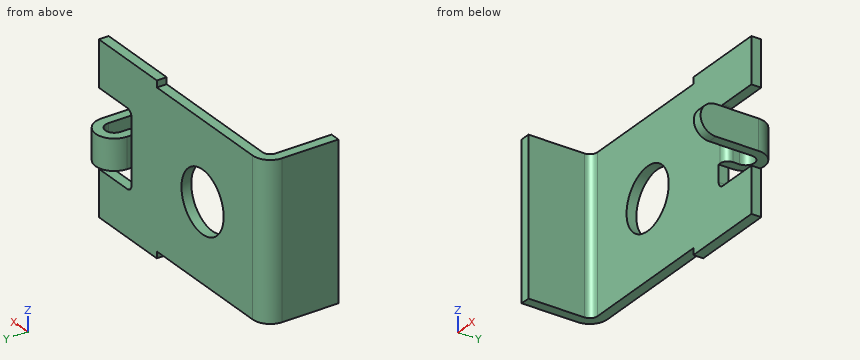
```python
from build123d import *

# Parameters (mm, degrees)
EXTRUDE_THIN1_DEPTH = 6.4135
SKETCH2_W           = 6.985
SKETCH2_H           = 0.8128
BOSS_EXTRUDE1_DEPTH = 6.9596
SKETCH3_W           = 3.937
SKETCH3_H           = 6.35
CUT_EXTRUDE1_DEPTH  = 23.027014146
EXTRUDE_THIN2_DEPTH = 1.27
FILLET1_RADIUS      = 1.27
FILLET1_LENGTH      = 0.8128
FILLET2_R           = 0.635
SKETCH5_R           = 2.54
CUT_EXTRUDE2_DEPTH  = 23.027014146
FILLET3_R           = 0.508


with BuildPart() as part:
    # Sketch1 → Extrude-Thin1 (new, symmetric)
    with BuildSketch(Plane.XY):
        with BuildLine():
            Line((0, 0), (0, 4.6482))
            ThreePointArc((0, 4.6482), (0.424050802, 5.671949198), (1.4478, 6.096))
            Line((1.4478, 6.096), (19.9898, 6.096))
            Line((19.9898, 6.096), (19.9898, 5.2832))
            Line((19.9898, 5.2832), (1.4478, 5.2832))
            ThreePointArc((1.4478, 5.2832), (0.998787194, 5.097212806), (0.8128, 4.6482))
            Line((0.8128, 4.6482), (0.8128, 0))
            Line((0.8128, 0), (0, 0))
        make_face()
    extrude(amount=EXTRUDE_THIN1_DEPTH, both=True)

    # Sketch2 → Boss-Extrude1 (add, symmetric)
    with BuildSketch(Plane.XY):
        with Locations((16.4973, 5.6896)):
            Rectangle(SKETCH2_W, SKETCH2_H)
    extrude(amount=BOSS_EXTRUDE1_DEPTH, both=True)

    # Sketch3 → Cut-Extrude1 (cut, through all)
    with BuildSketch(Plane(origin=(0, 6.096, 0), x_dir=(1, 0, 0), z_dir=(0, 1, 0))):
        with Locations((18.0213, 0)):
            Rectangle(SKETCH3_W, SKETCH3_H)
    extrude(amount=-CUT_EXTRUDE1_DEPTH, mode=Mode.SUBTRACT)

    # Sketch4 → Extrude-Thin2 (add, symmetric)
    with BuildSketch(Plane.XY):
        with BuildLine():
            Line((16.0528, 5.2832), (16.0528, 6.4516))
            ThreePointArc((16.0528, 6.4516), (17.6022, 8.001), (19.1516, 6.4516))
            Line((19.1516, 6.4516), (19.1516, 1.651))
            Line((19.1516, 1.651), (18.3388, 1.651))
            Line((18.3388, 1.651), (18.3388, 6.4516))
            ThreePointArc((18.3388, 6.4516), (17.6022, 7.1882), (16.8656, 6.4516))
            Line((16.8656, 6.4516), (16.8656, 5.2832))
            Line((16.8656, 5.2832), (16.0528, 5.2832))
        make_face()
    extrude(amount=EXTRUDE_THIN2_DEPTH, both=True)

    # Fillet1: full round fillet: the end face becomes a half cylinder, R = half its width
    fillet1_face = Plane((18.7452, 1.651, 0), x_dir=(-1, 0, 0), z_dir=(0, -1, 0))  # on the end face: x along it, z out of the body
    fillet1_slab = fillet1_face.offset(-FILLET1_RADIUS / 2) * Box(FILLET1_LENGTH, 2 * FILLET1_RADIUS, FILLET1_RADIUS, mode=Mode.PRIVATE)  # the body's end, R deep
    fillet1_round = Plane((18.7452, 2.921, 0), x_dir=(0, -1, 0), z_dir=(-1, 0, 0)) * Cylinder(FILLET1_RADIUS, FILLET1_LENGTH, mode=Mode.PRIVATE)  # its axis R under the face
    add(fillet1_slab - fillet1_round, mode=Mode.SUBTRACT)

    # Fillet2
    fillet2_edges = [part.edges().sort_by_distance(p)[0] for p in [
        (16.8656, 5.2832, 0),
    ]]
    fillet(fillet2_edges, radius=FILLET2_R)

    # Sketch5 → Cut-Extrude2 (cut, through all)
    with BuildSketch(Plane(origin=(0, 6.096, 0), x_dir=(1, 0, 0), z_dir=(0, 1, 0))):
        with Locations(Location((7.493, 0, 0), (0, 0, 270))):
            Circle(SKETCH5_R)
    extrude(amount=-CUT_EXTRUDE2_DEPTH, mode=Mode.SUBTRACT)

    # Fillet3
    fillet3_edges = [part.edges().sort_by_distance(p)[0] for p in [
        (16.0528, 5.6896, 3.175),
        (16.0528, 5.6896, -3.175),
    ]]
    fillet(fillet3_edges, radius=FILLET3_R)


solid = part.part
```
The listing builds one solid part. Answer for the finished solid, in the listing's coordinates (mm). Coordinates: 2 decimals unless noted, no trailing zeros. Loops run counter-clockwise (first coordinate to the right, second up) from the corner with the lowest first, then second, coordinate; pieces in that order, holes last. Notation, with made-up numbers: (50, 83.5) - (98, 83.5) arc R8 ccw to (98, 88.5) - close; hole circle Ø2 at (38, 34.25). An arc over 180 degrees is marked (long way). Use a Markdown table: item, result. Add a question column.
1) Find the intervals of material crossed by line 1 (X direction, y = 5.65, z = 0); line 2 (X direction, y = 5.5, z = 0); line 3 (X direction, y = 3, z = 0), in increasing order.
2) The part is cut by section B-B, the plane z = 4.5. Give the vertices of the cut face in (x, y) (3 decimals), and give its area (3 significant figures).
3) Given pin 1 (6 mm diameter, centred on x = 16, z = 5, fed in from +Y); pin 2 (6 mm diameter, centred on x = 5, z = 0, fed in from -Y); pin 3 (2 mm diameter, centred on y = 3.5, z = 0, fed in from +X); pin 4 (3 mm diameter, centred on x = 7.493, z = 0, fed in from -Y), each flat-ended and moving along its own axis, determine where each tip first touches the part or whether it passes through.
4) The part is cut by section D-D, the plane y = 5. Give the vertices of the cut face in (x, z).
5) The part is cut by section C-C, the plane x = 9. Give the vertices of the cut face in (y, z), and give its area (3 significant figures).
6) The part is cut by section A-A, the plane z = 0. Give the vertices of the cut face in (x, y) (3 decimals).
Here are the results:
| question | item | result |
|---|---|---|
| 1 | line 1 | x = 0.4 to 4.95, 10.03 to 16.81, 18.34 to 19.15 |
| 1 | line 2 | x = 0.28 to 4.95, 10.03 to 16.71, 18.34 to 19.15 |
| 1 | line 3 | x = 0 to 0.81, 18.34 to 19.15 |
| 2 | outline | (0, 0) - (0.813, 0) - (0.813, 4.648) arc R0.635 cw to (1.448, 5.283) - (19.99, 5.283) - (19.99, 6.096) - (1.448, 6.096) arc R1.448 ccw to (0, 4.648) - close |
| 2 | area | 20.2 mm^2 |
| 3 | pin 1 | stops at y = 6.1 |
| 3 | pin 2 | stops at y = 5.28 |
| 3 | pin 3 | stops at x = 19.15 |
| 3 | pin 4 | passes through |
| 4 | outline | (0.04, -6.41) - (0.92, -6.41) - (0.92, 6.41) - (0.04, 6.41) - close; (18.34, -1.27) - (19.15, -1.27) - (19.15, 1.27) - (18.34, 1.27) - close |
| 5 | outline | (5.28, -6.41) - (6.1, -6.41) - (6.1, -2.04) - (5.28, -2.04) - close; (5.28, 2.04) - (6.1, 2.04) - (6.1, 6.41) - (5.28, 6.41) - close |
| 5 | area | 7.10 mm^2 |
| 6 | outline | (0, 0) - (0.813, 0) - (0.813, 4.648) arc R0.635 cw to (1.448, 5.283) - (4.953, 5.283) - (4.953, 6.096) - (1.448, 6.096) arc R1.448 ccw to (0, 4.648) - close; (10.033, 5.283) - (16.231, 5.283) arc R0.635 ccw to (16.866, 5.918) - (16.866, 6.452) arc R0.737 cw to (18.339, 6.452) - (18.339, 1.651) - (19.152, 1.651) - (19.152, 6.452) arc R1.549 ccw to (16.053, 6.452) - (16.053, 6.096) - (10.033, 6.096) - close |
